Read the model definition and answer for the solid it produces. Units are mm, in the model's axes. A direction names the side the tool comes from. Give positions to 0.01 mm unless a question says otherwise; leave off trailing zeros. Loops run counter-clockwise (first coordinate to the right, second up) from the corner with the lowest first, then second, coordinate; pieces in that order, holes last.
(1) Find section C-C, the plane y = 1.45. State how many separate pieces and enclosed holes the cut face has, then the cut area to 3 significant figures.
(2) Which of the six approach directions +Z, -Z, +X, -X, +Y, -Y give full straight-line access (tool end or side, diameter ignored) to faces 1 (the face through (-19, 1, 17)), 2 (the face through (28.57, 0.99, 36.31)), 3 (the face through (45.78, 0.99, 4.55))?
(3) Find section D-D, the plane x = 67. Write down the section's boundary in (y, z).
(4) Straight lines are drawn through the part: probe 1 along X at (y, z) = (1, 3); probe 2 along Z at (x, y) = (0.5, 1.9); probe 3 along Z at (x, y) = (81.25, 0.7). For each, find the intervals that lie inside material, in ascending order.
(5) Determine the mould class of faces 4 (the face through (97.361, 0.986, 27.544)), 5 (the face through (43, 0, 19)), 6 (the face through (15, 1, 12.9)) for opening direction X: pulls with the +X half, pulls with the -X half, needs draft (parallel to the pull), parting line crosses it, or undercut.
(6) Find section A-A, the plane x = 13.5. Write down the section's boundary in (y, z), then the cut area to 3 significant figures.
(7) Find section B-B, the plane z = 15.5. Write down the section's boundary in (x, y).
(8) This flat-tipped pin is pushed along its axis until it touches: P1, Ø1, axis at x = 64, y = 0.5, coming from the -Z side. Where does it stop, or does it pass through?
```python
from build123d import *

# Parameters (mm, degrees)
SKETCH1_R           = 1.75
SKETCH1_R_2         = 1.5
SKETCH1_R_3         = 5
BOSS_EXTRUDE1_DEPTH = 2
FILLET1_R           = 1.5


with BuildPart() as part:
    # Sketch1 → Boss-Extrude1 (new body)
    with BuildSketch(Plane(origin=(0, 0, 0), x_dir=(1, 0, 0), z_dir=(0, 1, 0))):
        with BuildLine():
            Line((0, 0), (43, 0))
            Line((43, 0), (48.5, -9))
            Line((48.5, -9), (59.5, -12))
            Line((59.5, -12), (69.5, -12))
            Line((69.5, -12), (74.5, 2.5))
            Line((74.5, 2.5), (101.5, -0.5))
            Line((101.5, -0.5), (107, -9.5))
            Line((107, -9.5), (107, -24.5))
            Line((107, -24.5), (88, -30.5))
            Line((88, -30.5), (85.5, -34.5))
            ThreePointArc((85.5, -34.5), (82.533474843, -40.320323174), (76.870377201, -37.063674828))
            Line((76.870377201, -37.063674828), (74, -35))
            Line((74, -35), (63, -38))
            Line((63, -38), (53, -38))
            Line((53, -38), (42, -41))
            Line((42, -41), (34, -41))
            Line((34, -41), (23, -31.5))
            Line((23, -31.5), (-5, -31.5))
            Line((-5, -31.5), (-7, -40.5))
            Line((-7, -40.5), (-18, -40.5))
            Line((-18, -40.5), (-22, -35))
            Line((-22, -35), (-22, -24))
            Line((-22, -24), (-16, -10))
            Line((-16, -10), (-6, -8))
            Line((-6, -8), (0, 0))
        make_face()
        with Locations(Location((40.25, -36, 0), (0, 0, 270))):
            Circle(SKETCH1_R, mode=Mode.SUBTRACT)
        with Locations(Location((81.25, -36, 0), (0, 0, 270))):
            Circle(SKETCH1_R_2, mode=Mode.SUBTRACT)
        with Locations(Location((91, -16.5, 0), (0, 0, 270))):
            Circle(SKETCH1_R_3, mode=Mode.SUBTRACT)
        with Locations(Location((77, -0.5, 0), (0, 0, 270))):
            Circle(SKETCH1_R, mode=Mode.SUBTRACT)
        with Locations(Location((81, -9.5, 0), (0, 0, 270))):
            Circle(SKETCH1_R_2, mode=Mode.SUBTRACT)
        with Locations(Location((100, -2.5, 0), (0, 0, 270))):
            Circle(SKETCH1_R_2, mode=Mode.SUBTRACT)
        with Locations(Location((102, -19.75, 0), (0, 0, 270))):
            Circle(SKETCH1_R_2, mode=Mode.SUBTRACT)
        with Locations(Location((53, -19, 0), (0, 0, 270))):
            Circle(SKETCH1_R_2, mode=Mode.SUBTRACT)
        with Locations(Location((34.25, -19, 0), (0, 0, 270))):
            Circle(SKETCH1_R_2, mode=Mode.SUBTRACT)
        with Locations(Location((13.5, -12, 0), (0, 0, 270))):
            Circle(SKETCH1_R, mode=Mode.SUBTRACT)
        with BuildLine():
            Line((-16, -34.5), (-11.5, -34.5))
            ThreePointArc((-11.5, -34.5), (-10, -36), (-11.5, -37.5))
            Line((-11.5, -37.5), (-16, -37.5))
            ThreePointArc((-16, -37.5), (-17.5, -36), (-16, -34.5))
        make_face(mode=Mode.SUBTRACT)
    extrude(amount=BOSS_EXTRUDE1_DEPTH)

    # Fillet1
    fillet1_edges = [part.edges().sort_by_distance(p)[0] for p in [
        (0, 1, 0),
        (43, 1, 0),
        (48.5, 1, 9),
        (59.5, 1, 12),
        (69.5, 1, 12),
        (74.5, 1, -2.5),
        (101.5, 1, 0.5),
        (107, 1, 9.5),
        (107, 1, 24.5),
        (88, 1, 30.5),
        (85.5, 1, 34.5),
        (76.870377201, 1, 37.063674828),
        (74, 1, 35),
        (63, 1, 38),
        (53, 1, 38),
        (42, 1, 41),
        (34, 1, 41),
        (23, 1, 31.5),
        (-5, 1, 31.5),
        (-7, 1, 40.5),
        (-18, 1, 40.5),
        (-22, 1, 35),
        (-22, 1, 24),
        (-16, 1, 10),
        (-6, 1, 8),
    ]]
    fillet(fillet1_edges, radius=FILLET1_R)


solid = part.part
```
Entries:
1. separate pieces: 1
1. enclosed holes: 11
1. area: 3,870 mm2
2. face 1: -Z, -X, +Y, -Y
2. face 2: +Z, +Y, -Y
2. face 3: -Z, +Y, -Y
3. outline: (0, 12) - (2, 12) - (2, 36.91) - (0, 36.91) - close
4. probe 1: x = -2.25 to 44.83, 72.6 to 98.59, 101.41 to 103.03
4. probe 2: z = 0.02 to 31.5
4. probe 3: z = -1.75 to 8.02, 10.98 to 34.5, 37.5 to 40.51
5. face 4: pulls with the +X half
5. face 5: needs draft
5. face 6: undercut
6. outline: (0, 0) - (2, 0) - (2, 10.25) - (0, 10.25) - close; (0, 13.75) - (2, 13.75) - (2, 31.5) - (0, 31.5) - close
6. area: 56.0 mm2
7. outline: (-18.36, 0) - (86.1, 0) - (86.1, 2) - (-18.36, 2) - close; (95.9, 0) - (107, 0) - (107, 2) - (95.9, 2) - close
8. P1: stops at z = 12
